The model under review builds one solid part; all positions refer to its coordinate system, in mm. A direction names the side the tool comes from. Give positions to 0.01 mm unless a question says otherwise; leave off trailing zeros. Loops run counter-clockwise (first coordinate to the right, second up) from the corner with the lowest first, then second, coordinate; pieces in that order, holes last. Notation, with made-up numbers: (-16, 86.5) - (22, 86.5) arc R27 cw to (22, 115.5) - close; hole circle Ø8 at (-4, 2.25). An arc over 180 degrees is marked (long way). Answer as a JSON object with one key per item and string values.
from build123d import *

# Parameters (mm, degrees)
ESQUISSE2_R             = 1.75
ENL_V_MAT_EXTRU_1_DEPTH = 30.090204537
CHANFREIN1_SIZE         = 3
ESQUISSE4_OUTSIDE_W     = 53.542
ESQUISSE4_OUTSIDE_H     = 53.542
ENL_V_MAT_EXTRU_2_DEPTH = 30.090204537


with BuildPart() as part:
    # Esquisse1 → Révolution1 (revolve)
    with BuildSketch(Plane.XY, mode=Mode.PRIVATE) as r_volution1_sk:
        with BuildLine():
            Line((-5.9, -3.577708764), (-7.4209506, -4.5))
            Line((-7.4209506, -4.5), (-20, -4.5))
            Line((-20, -4.5), (-20, 0.1))
            Line((-20, 0.1), (-10, 0.1))
            Line((-10, 0.1), (-10, 6.9))
            Line((-10, 6.9), (-5, 6.9))
            Line((-5, 6.9), (-4.048749214, 5.587273915))
            ThreePointArc((-4.048749214, 5.587273915), (-6.7634037, 1.366151673), (-5.9, -3.577708764))
        make_face()
    revolve(r_volution1_sk.sketch.rotate(Axis((0, 18.9741444, 0), (0, -1, 0)), 270), axis=Axis((0, 18.9741444, 0), (0, -1, 0)))

    # Esquisse2 → Enlèv. mat.-Extru.1 (cut, through all)
    with BuildSketch(Plane(origin=(0, 0.1, 0), x_dir=(1, 0, 0), z_dir=(0, 1, 0))):
        with Locations(Location((-15, 0, 0), (0, 0, 270))):
            Circle(ESQUISSE2_R)
        with Locations(Location((15, 0, 0), (0, 0, 270))):
            Circle(ESQUISSE2_R)
    extrude(amount=-ENL_V_MAT_EXTRU_1_DEPTH, mode=Mode.SUBTRACT)

    # Chanfrein1
    chanfrein1_edges = [part.edges().sort_by_distance(p)[0] for p in [
        (-15, -4.5, -1.75),
        (15, -4.5, -1.75),
    ]]
    chamfer(chanfrein1_edges, length=CHANFREIN1_SIZE)

    # Esquisse4 outside → Enlèv. mat.-Extru.2 (cut, through all)
    with BuildSketch(Plane(origin=(0, 0.1, 0), x_dir=(1, 0, 0), z_dir=(0, 1, 0))):
        Rectangle(ESQUISSE4_OUTSIDE_W, ESQUISSE4_OUTSIDE_H)
        with BuildLine():
            ThreePointArc((-9.12, -7.799076868), (0, -12), (9.12, -7.799076868))
            ThreePointArc((9.12, -7.799076868), (11.797195727, -5.758231957), (15.076923077, -4.999408249))
            ThreePointArc((15.076923077, -4.999408249), (20, 0), (15.076923077, 4.999408249))
            ThreePointArc((15.076923077, 4.999408249), (11.797195727, 5.758231957), (9.12, 7.799076868))
            ThreePointArc((9.12, 7.799076868), (0, 12), (-9.12, 7.799076868))
            ThreePointArc((-9.12, 7.799076868), (-11.797195727, 5.758231957), (-15.076923077, 4.999408249))
            ThreePointArc((-15.076923077, 4.999408249), (-20, 0), (-15.076923077, -4.999408249))
            ThreePointArc((-15.076923077, -4.999408249), (-11.797195727, -5.758231957), (-9.12, -7.799076868))
        make_face(mode=Mode.SUBTRACT)
    extrude(amount=-ENL_V_MAT_EXTRU_2_DEPTH, mode=Mode.SUBTRACT)


solid = part.part
Q1. The part is to be moulded in two halves that separate along X. For faces 1 (the face through (16.735, -0.689, -0.228)), 2 (the face through (20, -2, 0)), 3 (the face through (0, -2, -12)), 4 (the face through (-20, -2, 0)), say which applies: +X half, -X half, draft (parallel to the pull), parting line (faces both ways), or undercut.
Results:
{"face 1": "undercut", "face 2": "+X half", "face 3": "parting line", "face 4": "-X half"}
Q2. Consider section C-C, the plane y = -0.75. State the section outline as (x, z) points.
Results:
{"outline": "(-15.08, -5) arc R8 cw to (-9.12, -7.8) arc R12 ccw to (9.12, -7.8) arc R8 cw to (15.08, -5) arc R5 ccw to (15.08, 5) arc R8 cw to (9.12, 7.8) arc R12 ccw to (-9.12, 7.8) arc R8 cw to (-15.08, 5) arc R5 ccw to start; hole circle Ø3.5 at (-15, 0); hole circle Ø13.72 at (0, 0); hole circle Ø3.5 at (15, 0)"}
Q3. For faces 5 (the face through (16.88, -1.646, -0.247)), 6 (the face through (7.3, 0.1, -7.2)), list the 3-axis set-ups (+Z, -Z, +X, -X, +Y, -Y) from which the entire face can be reached by the end or side of a thin tool; tool diameter is ignored.
Results:
{"face 5": "-Y", "face 6": "+Y"}
Q4. Consider section A-A, the plane x = 0. State the section outline as (y, z) points, plus the area to 3 significant figures.
Results:
{"outline": "(-4.5, -12) - (0.1, -12) - (0.1, -10) - (6.9, -10) - (6.9, -5) - (5.59, -4.05) arc R6.9 cw to (-3.58, -5.9) - (-4.5, -7.42) - close; (-4.5, 7.42) - (-3.58, 5.9) arc R6.9 cw to (5.59, 4.05) - (6.9, 5) - (6.9, 10) - (0.1, 10) - (0.1, 12) - (-4.5, 12) - close", "area": "108 mm^2"}
Q5. Consider section B-B, the plane z = 0. State the section outline as (x, y) points, plus the area to 3 significant figures.
Results:
{"outline": "(-20, -4.5) - (-19.75, -4.5) - (-16.75, -1.5) - (-16.75, 0.1) - (-20, 0.1) - close; (-13.25, -1.5) - (-10.25, -4.5) - (-7.42, -4.5) - (-5.9, -3.58) arc R6.9 cw to (-4.05, 5.59) - (-5, 6.9) - (-10, 6.9) - (-10, 0.1) - (-13.25, 0.1) - close; (4.05, 5.59) arc R6.9 cw to (5.9, -3.58) - (7.42, -4.5) - (10.25, -4.5) - (13.25, -1.5) - (13.25, 0.1) - (10, 0.1) - (10, 6.9) - (5, 6.9) - close; (16.75, -1.5) - (19.75, -4.5) - (20, -4.5) - (20, 0.1) - (16.75, 0.1) - close", "area": "131 mm^2"}
Q6. To check wall thickness, follow probe 1 along X at (y, z) = (2, 1); probe 2 along Z at (x, y) = (5.5, 2); probe 3 along X at (y, z) = (0.25, -4). State the ranges of each line that lie inside material, in increasing order. Write a range as [from, to].
Results:
{"probe 1": "x = [-9.95, -6.53], [6.53, 9.95]", "probe 2": "z = [-8.35, -3.66], [3.66, 8.35]", "probe 3": "x = [-9.17, -5.62], [5.62, 9.17]"}
Q7. Consider section D-D, the plane z = -9.5. State the section outline as (x, y) points.
Results:
{"outline": "(-7.33, -4.5) - (7.33, -4.5) - (7.33, 0.1) - (3.12, 0.1) - (3.12, 6.9) - (-3.12, 6.9) - (-3.12, 0.1) - (-7.33, 0.1) - close"}
Q8. Clearance check with flat-ended pins moving along their axes: pin 1 Ø1 at (y, z) = (5.5, -9) entering from -X; pin 2 Ø4 at (x, z) = (15, -5.5) entering from +Y; pin 3 Ø1 at (y, z) = (4.5, 7.5) entering from -X. State where each tip first meets the part, or that it passes through.
Results:
{"pin 1": "stops at x = -5.27", "pin 2": "stops at y = 0.1", "pin 3": "stops at x = -7.14"}
